from build123d import *

# Parameters (mm, degrees)
SKETCH1_W                = 95.885
SKETCH1_H                = 90.17
SKETCH1_R                = 3.175
BOSS_EXTRUDE1_DEPTH      = 1.6
BOSS_EXTRUDE2_DEPTH      = 7.95
BOSS_EXTRUDE2_DEPTH_BACK = 0.4
SKETCH1_3_R              = 3.175


with BuildPart() as part:
    # Sketch1 → Boss-Extrude1 (new body)
    with BuildSketch(Plane.XY):
        Rectangle(SKETCH1_W, SKETCH1_H)
        with Locations((42.8625, -40.005)):
            Circle(SKETCH1_R, mode=Mode.SUBTRACT)
        with Locations((-42.8625, -36.195)):
            Circle(SKETCH1_R, mode=Mode.SUBTRACT)
        with Locations((-42.8625, 37.465)):
            Circle(SKETCH1_R, mode=Mode.SUBTRACT)
        with Locations((42.8625, 40.005)):
            Circle(SKETCH1_R, mode=Mode.SUBTRACT)
    extrude(amount=BOSS_EXTRUDE1_DEPTH)

    # Sketch1<3> → Boss-Extrude2 (add, two sides: drawn at the far end of the back side and taken through both)
    with BuildSketch(Plane.XY.offset(-BOSS_EXTRUDE2_DEPTH_BACK)):
        with Locations((42.8625, 40.005)):
            Circle(SKETCH1_3_R)
        with Locations((-42.8625, -36.195)):
            Circle(SKETCH1_3_R)
        with Locations((42.8625, -40.005)):
            Circle(SKETCH1_3_R)
        with Locations((-42.8625, 37.465)):
            Circle(SKETCH1_3_R)
    extrude(amount=BOSS_EXTRUDE2_DEPTH + BOSS_EXTRUDE2_DEPTH_BACK)


solid = part.part
Model file for the job. Use its own axes, mm. A direction names the side the tool comes from. Give positions to 0.01 mm unless a question says otherwise; leave off trailing zeros. Loops run counter-clockwise (first coordinate to the right, second up) from the corner with the lowest first, then second, coordinate; pieces in that order, holes last. Notation, with made-up numbers: (38, 85) - (74, 85) arc R24 ccw to (74, 122) - close; hole circle Ø10 at (-12.75, 32). An arc over 180 degrees is marked (long way). Use one line per item in the form item = value.
(1) Cut at A-A (y = 13). Give the cut face in (x, z), then the cut area to 3 significant figures.
Determined:
outline = (-47.94, 0) - (47.94, 0) - (47.94, 1.6) - (-47.94, 1.6) - close
area = 153 mm^2
(2) Cut at B-B (x = -34). Give the cut face in (y, z) (3 decimals), then the cut area to 3 significant figures.
Determined:
outline = (-45.085, 0) - (45.085, 0) - (45.085, 1.6) - (-45.085, 1.6) - close
area = 144 mm^2
(3) Drill centre lines: L1, parallel to Z at x = -32.5, y = 17.5; L2, parallel to X at y = -40, z = 2.25; L3, parallel to X at y = 37.5, z = 2. Where is each one in solid material? Low to high.
Determined:
L1 = 0 to 1.6
L2 = 39.69 to 46.04
L3 = -46.04 to -39.69, 40.91 to 44.81
(4) Cut at C-C (z = 4.25). Count the separate pieces of the cut face and the enclosed holes in it, then the cut area to 3 significant figures.
Determined:
separate_pieces = 4
enclosed_holes = 0
area = 127 mm^2
(5) Drop flat-ended pins along their axis: P1, Ø12, axis at x = 30, y = -15, coming from the -Z side; P2, Ø6, axis at x = -19.5, y = -2, coming from the +Z side. Give the stop position or say it passes through.
Determined:
P1 = 0
P2 = 1.6
(6) 3-axis set-ups, long thin cutter, end or side, ignore diameter. For faces 1 (the face through (-43, -36, 7.95)), 2 (the face through (-45.203, 39.611, 4.731)), 3 (the face through (-43.551, -39.294, -0.203)): which of +Z, -Z, +X, -X, +Y, -Y reach the whole face in a straight line?
Determined:
face_1 = +Z, +X, -X, +Y, -Y
face_2 = +Z
face_3 = -Z
(7) Pull direction X, two halves, no side cores. Call faces 4 (the face through (45.795, -41.221, 4.731)), 5 (the face through (43, 40, 7.95)): pulls with the +X half, pulls with the -X half, needs draft (parallel to the pull), parting line crosses it, or undercut.
Determined:
face_4 = undercut
face_5 = needs draft
